from build123d import *

# Parameters (mm, degrees)
BOSS_EXTRUDE1_DEPTH = 12
CUT_EXTRUDE1_REACH  = 14
SKETCH2_R           = 3.5
FILLET1_R           = 10
CUT_EXTRUDE2_REACH  = 14
SKETCH3_R           = 16.5
SKETCH4_W           = 20
SKETCH4_H           = 20
BOSS_EXTRUDE2_DEPTH = 12
FILLET2_R           = 5


with BuildPart() as part:
    # Sketch1 → Boss-Extrude1 (new body)
    with BuildSketch(Plane.XY):
        Polygon((-209, 0), (209, 0), (234, 43.301270189), (25, 405.299888971), (-25, 405.299888971), (-234, 43.301270189), align=None)
    extrude(amount=BOSS_EXTRUDE1_DEPTH)

    # Sketch2 → Cut-Extrude1 (cut, up to next)
    with BuildSketch(Plane.XY.offset(12), mode=Mode.PRIVATE) as cut_extrude1_sk1:
        with Locations((211.107695155, 27.650635095)):
            Circle(SKETCH2_R)
    cut_extrude1_tool1 = extrude(cut_extrude1_sk1.sketch, amount=-CUT_EXTRUDE1_REACH, mode=Mode.PRIVATE) & part.part
    add(cut_extrude1_tool1.solids().sort_by_distance((211.107695, 27.650635, 12))[0], mode=Mode.SUBTRACT)
    # Sketch2 → Cut-Extrude1 (cut, up to next)
    with BuildSketch(Plane.XY.offset(12), mode=Mode.PRIVATE) as cut_extrude1_sk2:
        with Locations((0, 393.299888971)):
            Circle(SKETCH2_R)
    cut_extrude1_tool2 = extrude(cut_extrude1_sk2.sketch, amount=-CUT_EXTRUDE1_REACH, mode=Mode.PRIVATE) & part.part
    add(cut_extrude1_tool2.solids().sort_by_distance((0, 393.299889, 12))[0], mode=Mode.SUBTRACT)
    # Sketch2 → Cut-Extrude1 (cut, up to next)
    with BuildSketch(Plane.XY.offset(12), mode=Mode.PRIVATE) as cut_extrude1_sk3:
        with Locations((-211.107695155, 27.650635095)):
            Circle(SKETCH2_R)
    cut_extrude1_tool3 = extrude(cut_extrude1_sk3.sketch, amount=-CUT_EXTRUDE1_REACH, mode=Mode.PRIVATE) & part.part
    add(cut_extrude1_tool3.solids().sort_by_distance((-211.107695, 27.650635, 12))[0], mode=Mode.SUBTRACT)

    # Fillet1
    fillet1_edges = [part.edges().sort_by_distance(p)[0] for p in [
        (-25, 405.299888971, 6),
        (25, 405.299888971, 6),
        (234, 43.301270189, 6),
        (209, 0, 6),
        (-209, 0, 6),
        (-234, 43.301270189, 6),
    ]]
    fillet(fillet1_edges, radius=FILLET1_R)

    # Sketch3 → Cut-Extrude2 (cut, up to next)
    with BuildSketch(Plane.XY.offset(12), mode=Mode.PRIVATE) as cut_extrude2_sk1:
        with Locations((-40, 80)):
            Circle(SKETCH3_R)
    cut_extrude2_tool1 = extrude(cut_extrude2_sk1.sketch, amount=-CUT_EXTRUDE2_REACH, mode=Mode.PRIVATE) & part.part
    add(cut_extrude2_tool1.solids().sort_by_distance((-40, 80, 12))[0], mode=Mode.SUBTRACT)
    # Sketch3 → Cut-Extrude2 (cut, up to next)
    with BuildSketch(Plane.XY.offset(12), mode=Mode.PRIVATE) as cut_extrude2_sk2:
        with Locations((40, 80)):
            Circle(SKETCH3_R)
    cut_extrude2_tool2 = extrude(cut_extrude2_sk2.sketch, amount=-CUT_EXTRUDE2_REACH, mode=Mode.PRIVATE) & part.part
    add(cut_extrude2_tool2.solids().sort_by_distance((40, 80, 12))[0], mode=Mode.SUBTRACT)
    # Sketch3 → Cut-Extrude2 (cut, up to next)
    with BuildSketch(Plane.XY.offset(12), mode=Mode.PRIVATE) as cut_extrude2_sk3:
        with Locations((-120, 80)):
            Circle(SKETCH3_R)
    cut_extrude2_tool3 = extrude(cut_extrude2_sk3.sketch, amount=-CUT_EXTRUDE2_REACH, mode=Mode.PRIVATE) & part.part
    add(cut_extrude2_tool3.solids().sort_by_distance((-120, 80, 12))[0], mode=Mode.SUBTRACT)
    # Sketch3 → Cut-Extrude2 (cut, up to next)
    with BuildSketch(Plane.XY.offset(12), mode=Mode.PRIVATE) as cut_extrude2_sk4:
        with Locations((120, 80)):
            Circle(SKETCH3_R)
    cut_extrude2_tool4 = extrude(cut_extrude2_sk4.sketch, amount=-CUT_EXTRUDE2_REACH, mode=Mode.PRIVATE) & part.part
    add(cut_extrude2_tool4.solids().sort_by_distance((120, 80, 12))[0], mode=Mode.SUBTRACT)

    # Sketch4 → Boss-Extrude2 (add)
    with BuildSketch(Plane.XY.offset(12)):
        with Locations((0, 415.299888971)):
            Rectangle(SKETCH4_W, SKETCH4_H)
        Polygon((226.5, 30.310889132), (243.820508076, 20.310889132), (233.820508076, 2.990381057), (216.5, 12.990381057), align=None)
        Polygon((-226.5, 30.310889132), (-243.820508076, 20.310889132), (-233.820508076, 2.990381057), (-216.5, 12.990381057), align=None)
    extrude(amount=-BOSS_EXTRUDE2_DEPTH)

    # Fillet2
    fillet2_edges = [part.edges().sort_by_distance(p)[0] for p in [
        (216.5, 12.990381057, 6),
        (226.5, 30.310889132, 6),
        (-226.5, 30.310889132, 6),
        (-216.5, 12.990381057, 6),
        (10, 405.299888971, 6),
        (-10, 405.299888971, 6),
    ]]
    fillet(fillet2_edges, radius=FILLET2_R)


solid = part.part
Input: part model. Units: mm. Frame: model coordinates. A direction names the side the tool comes from. Give positions to 0.01 mm unless a question says otherwise; leave off trailing zeros. Write each loop counter-clockwise with the first axis right and the second up, starting at its lowest first coordinate (ties: lowest second). Pieces come first, ordered by that corner, then holes.
Q1. Section D-D, the plane z = 9.5. State how many separate pieces and enclosed holes the cut face has, plus the area to 3 significant figures.
Q2. Section C-C, the plane x = -40. Output: boundary loops of the cut face in (y, z).
Q3. Section B-B, the plane y = 249. Output: boundary loops of the cut face in (x, z).
Q4. Section A-A, the plane x = -120. Output: boundary loops of the cut face in (y, z).
Q5. Pull-direction query (Y, two-part tool) for faces 1 (the face through (107.84, 91.15, 6.08)), 2 (the face through (238.89, 11.77, 6.08)), 3 (the face through (-3, 168, 12)); classes: pulls with the +Y half, pulls with the -Y half, needs draft (parallel to the pull), parting line crosses it, or undercut.
Q6. Set-up query: faces 4 (the face through (10, 418, 6)), 5 (the face through (-227.416, 6.688, 6.084)), 6 (the face through (-238.89, 11.77, 6.08)). Return all of +Z, -Z, +X, -X, +Y, -Y with unobstructed straight access to the full face (end or side cutting, diameter ignored); none if empty.
Q7. First-contact query: P1, Ø5, axis at y = 109.5, z = 7.5, coming from the +X side; P2, Ø5, axis at x = 193.5, z = 4, coming from the +Y side; P3, Ø8, axis at x = 0, y = 393.3, coming from the +Z side; P4, Ø1.5, axis at y = 352.5, z = 9.5, coming from the +X side. Flat tips, straight axial feed; report the tip coordinate or a pass-through.
Q8. Material intervals for probe 1 along Y at (x, z) = (0, 4.25); probe 2 along Y at (x, z) = (40, 5.75); probe 3 along Y at (x, z) = (86, 4.75), sorted ascending.
Filled in:
1. separate pieces: 1
1. enclosed holes: 7
1. area: 111,000 mm2
2. outline: (0, 0) - (63.5, 0) - (63.5, 12) - (0, 12) - close; (96.5, 0) - (379.32, 0) - (379.32, 12) - (96.5, 12) - close
3. outline: (-115.24, 0) - (115.24, 0) - (115.24, 12) - (-115.24, 12) - close
4. outline: (0, 0) - (63.5, 0) - (63.5, 12) - (0, 12) - close; (96.5, 0) - (240.76, 0) - (240.76, 12) - (96.5, 12) - close
5. face 1: undercut
5. face 2: pulls with the -Y half
5. face 3: needs draft
6. face 4: +Z, -Z, +X, +Y
6. face 5: +Z, -Z, -Y
6. face 6: +Z, -Z, -X, -Y
7. P1: stops at x = 197.22
7. P2: stops at y = 117.78
7. P3: stops at z = 12
7. P4: stops at x = 55.92
8. probe 1: y = 0 to 389.8, 396.8 to 425.3
8. probe 2: y = 0 to 63.5, 96.5 to 379.32
8. probe 3: y = 0 to 299.64
